Can you work these out from the drawing? Everything is in mm from the part's minimum corner. A direction names the side the tool comes from. Coordinates: 2 decimals unless noted, no trailing zeros. Order: outer loops, then holes, each group sorted by start corner. A loop starts at its lowest first (then second) coordinate and runs counter-clockwise, first axis right, second up. Notation, with made-up numbers: (-16.5, 60.25) -> (1.5, 60.25) arc R17 ccw to (1.5, 64.25) -> close; hole circle Ø3 at (34, 66.25). An arc over 180 degrees is marked (long way). Return JSON: item names as keys, results as strings. Group by question number.
1) Thinking about a two-plate mould opening in Y: for the marked faces 3, 4, 5 and 6, which applies, +Y half, -Y half, draft (parallel to the pull), parting line (faces both ways), or undercut?
2) For pin 1 (5 mm diameter, centred on y = 5.5, z = 2.5, fed in from +X); pin 2 (5 mm diameter, centred on x = 11.11, y = 11.11, fed in from +Z); pin 3 (8 mm diameter, centred on x = 14.5, y = 11.5, fed in from +Z); pin 4 (4 mm diameter, centred on x = 6, z = 10.5, fed in from -Y) (1 decimal), each with a flat end and sliding along its axis, tell me the tip position at first contact or that it passes through.
3) If I drill on probe 1 along Y at (x, z) = (11.25, 8.5) (1 decimal); probe 2 along Z at (x, y) = (3.5, 15.5) (1 decimal); probe 3 along Z at (x, y) = (7.25, 17) (1 decimal), over which ranges is the centre line in solid material (lowest first)? Write a range as from..to.
4) If we section it at B-B, the plane y = 13.75: Please give me the cut outline in (x, z) (1 decimal), then the cut area to 3 significant figures.
5) For the marked faces 1 and 2, which set-ups out of +Z, -Z, +X, -X, +Y, -Y let a thin tool reach every point of the face, with its end or its side?
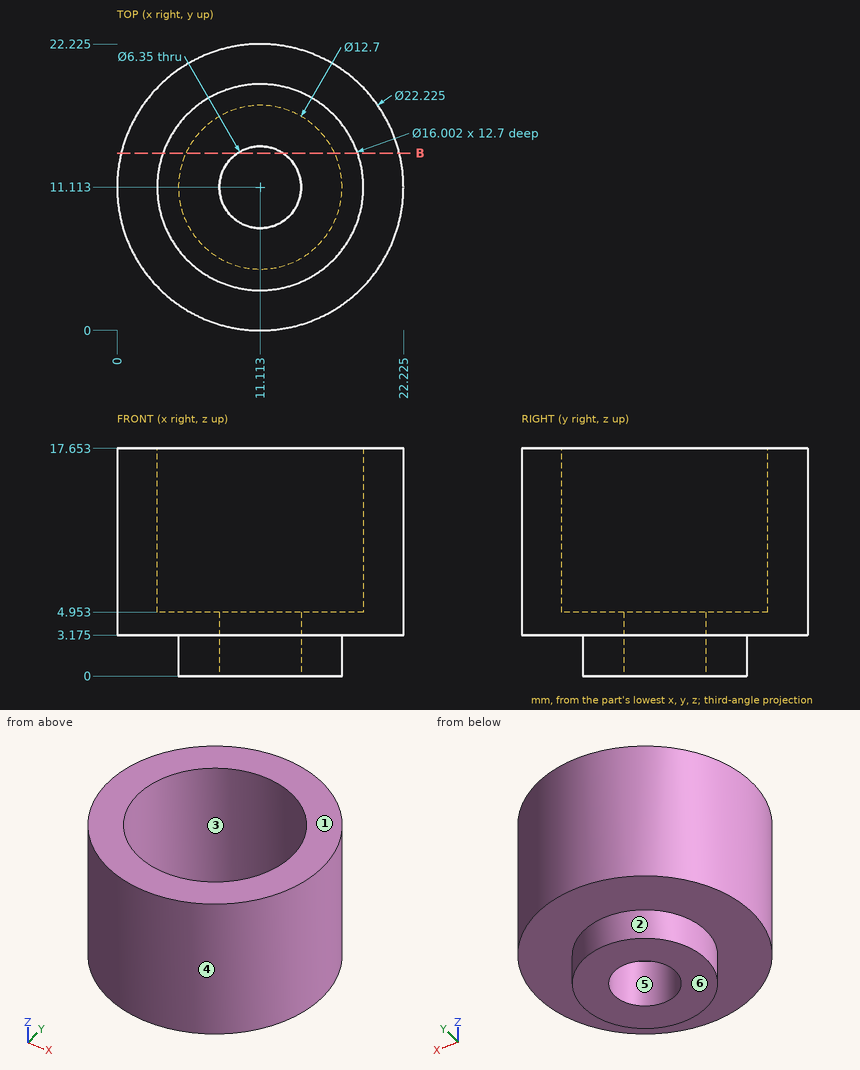
Result sheet:
{
 "1": {"face 3": "undercut", "face 4": "parting line", "face 5": "undercut", "face 6": "draft"},
 "2": {"pin 1": "stops at x = 21.75", "pin 2": "passes through", "pin 3": "stops at z = 4.95", "pin 4": "stops at y = 0.4"},
 "3": {"probe 1": "y = 0..3.1, 19.1..22.2", "probe 2": "z = 3.2..17.7", "probe 3": "z = 3.2..5"},
 "4": {"outline": "(0.3, 3.2) -> (5.3, 3.2) -> (5.3, 0) -> (9.3, 0) -> (9.3, 5) -> (3.6, 5) -> (3.6, 17.7) -> (0.3, 17.7) -> close; (12.9, 0) -> (16.9, 0) -> (16.9, 3.2) -> (21.9, 3.2) -> (21.9, 17.7) -> (18.7, 17.7) -> (18.7, 5) -> (12.9, 5) -> close", "area": "140 mm2"},
 "5": {"face 1": "+Z, +X, -X, +Y, -Y", "face 2": "-Z"}
}
